```python
from build123d import *

# Parameters (mm, degrees)
SKETCH1_W           = 50.8
SKETCH1_H           = 86.36
BOSS_EXTRUDE1_DEPTH = 5.08
SKETCH2_W           = 7.366
SKETCH2_H           = 5.08
CUT_EXTRUDE1_DEPTH  = 5.08
SKETCH6_W           = 7.365
SKETCH6_H           = 5.08
CUT_EXTRUDE2_DEPTH  = 5.08


with BuildPart() as part:
    # Sketch1 → Boss-Extrude1 (new body)
    with BuildSketch(Plane.XY):
        with Locations((-25.4, 43.18)):
            Rectangle(SKETCH1_W, SKETCH1_H)
    extrude(amount=BOSS_EXTRUDE1_DEPTH)

    # Sketch2 → Cut-Extrude1 (cut)
    with BuildSketch(Plane(origin=(0, 86.36, 0), x_dir=(1, 0, 0), z_dir=(0, 1, 0))):
        with Locations((-47.117, -2.54)):
            Rectangle(SKETCH2_W, SKETCH2_H)
        with Locations((-3.683, -2.54)):
            Rectangle(SKETCH2_W, SKETCH2_H)
    extrude(amount=-CUT_EXTRUDE1_DEPTH, mode=Mode.SUBTRACT)

    # Sketch6 → Cut-Extrude2 (cut)
    with BuildSketch(Plane(origin=(0, 0, 0), x_dir=(-1, 0, 0), z_dir=(0, -1, 0))):
        with Locations((47.1175, -2.54)):
            Rectangle(SKETCH6_W, SKETCH6_H)
        with Locations((3.6825, -2.54)):
            Rectangle(SKETCH6_W, SKETCH6_H)
    extrude(amount=-CUT_EXTRUDE2_DEPTH, mode=Mode.SUBTRACT)


solid = part.part
```
Part model, mm, in its own coordinate system. A direction names the side the tool comes from. Round coordinates to 2 decimals unless told otherwise and drop trailing zeros. Loops run counter-clockwise (first coordinate to the right, second up) from the corner with the lowest first, then second, coordinate; pieces in that order, holes last.
Item 1: 3-axis set-ups, long thin cutter, end or side, ignore diameter. For faces 1 (the face through (-43.435, 3, 3)), 2 (the face through (-7.365, 3, 3)), 3 (the face through (-4, 81.28, 3)), 4 (the face through (-43.434, 84, 3)): which of +Z, -Z, +X, -X, +Y, -Y reach the whole face in a straight line?
Item 2: Cut at B-B, the plane x = -45. Give the cut face in (y, z).
Item 3: Drop flat-ended pins along their axis: P1, Ø2.5, axis at x = -3, z = 3.5, coming from the -Y side; P2, Ø2.5, axis at y = 3.5, z = 2.5, coming from the +X side (3 decimals); P3, Ø1.5, axis at x = -47.5, z = 1.5, coming from the +Y side. Give the stop position or say it passes through.
Item 4: Cut at A-A, the plane z = 3.65. Give the cut face in (x, y) (3 decimals), then the cut area to 3 significant figures.
Item 5: Drill centre line: line 1 (Y direction, x = -44.5, z = 2.5). Where is it in solid material? Low to high.
A:
1. face 1: +Z, -Z, -X, -Y
1. face 2: +Z, -Z, +X, -Y
1. face 3: +Z, -Z, +X, +Y
1. face 4: +Z, -Z, -X, +Y
2. outline: (5.08, 0) - (81.28, 0) - (81.28, 5.08) - (5.08, 5.08) - close
3. P1: stops at y = 5.08
3. P2: stops at x = -7.365
3. P3: stops at y = 81.28
4. outline: (-50.8, 5.08) - (-43.435, 5.08) - (-43.435, 0) - (-7.365, 0) - (-7.365, 5.08) - (0, 5.08) - (0, 81.28) - (-7.366, 81.28) - (-7.366, 86.36) - (-43.434, 86.36) - (-43.434, 81.28) - (-50.8, 81.28) - close
4. area: 4,240 mm2
5. line 1: y = 5.08 to 81.28
